Autodesk Inventor part; units mm, degrees
ref_plane "YZ Plane" through (0, 0, 0) normal (1, 0, 0) x (0, 1, 0)
ref_plane "XZ Plane" through (0, 0, 0) normal (0, 1, 0) x (-1, 0, 0)
ref_plane "XY Plane" through (0, 0, 0) normal (0, 0, 1) x (1, 0, 0)
sketch "Sketch1" plane through (0, 0, 0) normal (0, 0, 1) x (1, 0, 0)
  line L0 (-56.0804, 17.6748) -> (23.9196, 17.6748)
  line L1 (23.9196, 17.6748) -> (23.9196, -24.3252)
  line L2 (23.9196, -24.3252) -> (-56.0804, -24.3252)
  line L3 (-56.0804, -24.3252) -> (-56.0804, 17.6748)
  line L4 (-57.3304, 19.1748) -> (25.4196, 19.1748)
  line L5 (25.4196, 19.1748) -> (25.4196, -25.8252)
  line L6 (25.4196, -25.8252) -> (-57.3304, -25.8252)
  line L7 (-57.3304, -25.8252) -> (-57.3304, 19.1748)
  point P0 (0, 0)
  dimension "d0" = 80
  dimension "d1" = 42
  dimension "d2" = 1.5
  dimension "d3" = 1.5
  dimension "d4" = 1.25
  dimension "d5" = 1.5
extrude "Extrusion1" add sketch "Sketch1" along normal blind 24
sketch "Sketch2" plane through (0, 0, 0) normal (0, 0, -1) x (-1, 0, 0)
  line L0 (-25.4196, -25.8252) -> (-25.4196, 19.1748)
  line L1 (57.3304, -25.8252) -> (-25.4196, -25.8252)
  line L2 (-25.4196, 19.1748) -> (57.3304, 19.1748)
  line L3 (57.3304, 19.1748) -> (57.3304, -25.8252)
  line L4 (57.3304, -25.8252) -> (-25.4196, -25.8252)
  line L5 (-25.4196, -25.8252) -> (-25.4196, 19.1748)
  point P0 (0, 0)
extrude "Extrusion2" add sketch "Sketch2" along normal blind 1.2
fillet "Fillet1" radius 2 4 edges at (-57.3304, 19.1748, 11.4) (-57.3304, -25.8252, 11.4) (25.4196, -25.8252, 11.4) (25.4196, 19.1748, 11.4)
sketch "Sketch3" plane through (0, 0, 0) normal (0, 0, 1) x (1, 0, 0)
  line L0 (-56.0804, 17.6748) -> (23.9196, 17.6748)
  line L1 (-45.0804, 17.6748) -> (17.9196, 17.6748)
  line L2 (17.9196, 17.6748) -> (17.9196, -24.8955)
  line L3 (17.9196, -24.8955) -> (-45.0804, -24.8955)
  line L4 (-45.0804, -24.8955) -> (-45.0804, 17.6748)
  line L5 (23.9196, 17.6748) -> (23.9196, -24.3252)
  point P0 (0, 0)
  point P1 (17.9196, 17.6748)
  dimension "d11" = 6
  dimension "d12" = 69
extrude "Extrusion3" cut sketch "Sketch3" against normal blind 1.2
chamfer "Chamfer1" distance 1.2 angle 45 2 edges at (-45.0804, -3.3252, 0) (17.9196, -3.3252, 0)
sketch "Sketch4" plane through (-57.3304, -23.8252, 24) normal (-1, 0, 0) x (0, 0, 1)
  line L0 (-15, 14.5) -> (-20, 14.5)
  line L1 (-20, 14.5) -> (-20, 4.5)
  line L2 (-20, 4.5) -> (-15, 4.5)
  line L3 (-15, 4.5) -> (-15, 14.5)
  line L4 (-24, -0.5) -> (-24, 41.5)
  line L5 (-24, -0.5) -> (0, -0.5)
  point P0 (-24, 23.8252)
  dimension "d18" = 4
  dimension "d19" = 5
  dimension "d20" = 10
  dimension "d21" = 5
extrude "Extrusion4" cut sketch "Sketch4" against normal blind 1.5
sketch "Sketch5" plane through (-57.3304, -23.8252, 24) normal (-1, 0, 0) x (0, 0, 1)
  line L0 (0, 43) -> (-25.2, 43)
  line L1 (-25.2, -2) -> (0, -2)
  line L2 (0, 41) -> (0, 0)
  point P0 (-24, 23.8252)
  point P1 (-3, 33)
  point P2 (-3, 8)
  dimension "d24" = 10
  dimension "d25" = 10
  dimension "d26" = 3
  dimension "d27" = 3
hole "Hole1" at (-57.3304, 9.1748, 21) at (-57.3304, -15.8252, 21) direction (1, 0, 0) diameter 2 depth 10 tip angle 179 countersink diameter 4 countersink angle 90
sketch "Sketch6" plane through (25.4196, -23.8252, 24) normal (1, 0, 0) x (0, 0, -1)
  circle A0 centre (3, 8) radius 1
  circle A1 centre (3, 33) radius 1
  point P0 (24, 23.8252)
hole "Hole2" at (25.4196, -15.8252, 21) at (25.4196, 9.1748, 21) direction (-1, 0, 0) diameter 2 depth 10 tip angle 179 countersink diameter 4 countersink angle 90
sketch "Sketch7" plane through (0, 0, -1.2) normal (0, 0, -1) x (-1, 0, 0)
  line L0 (45.0804, -24.8955) -> (-17.9196, -24.8955)
  line L1 (-17.9196, -24.3252) -> (-17.9196, 17.6748)
  line L2 (45.0804, -24.8955) -> (-17.9196, -24.8955)
  line L3 (-17.9196, -24.8955) -> (-17.9196, -24.3252)
  line L4 (-17.9196, -24.3252) -> (45.0804, -24.3252)
  line L5 (45.0804, -24.3252) -> (45.0804, -24.8955)
  point P0 (0, 0)
extrude "Extrusion5" add sketch "Sketch7" against normal blind 1.5
sketch "Sketch8" plane through (0, 0, -1.2) normal (0, 0, -1) x (-1, 0, 0)
  line L0 (-17.9196, -24.3252) -> (-17.9196, 17.6748)
  line L1 (-23.9196, -24.3252) -> (56.0804, -24.3252)
  line L2 (-17.9196, 17.6748) -> (41.0804, 17.6748)
  line L3 (41.0804, 17.6748) -> (41.0804, -24.3252)
  line L4 (41.0804, -24.3252) -> (-17.9196, -24.3252)
  line L5 (-17.9196, -24.3252) -> (-17.9196, 17.6748)
  line L6 (-23.9196, 17.6748) -> (-23.9196, -24.3252)
  line L7 (46.2804, -24.3252) -> (56.0804, -24.3252)
  line L8 (41.0804, 17.6748) -> (56.0804, 17.6748)
  line L9 (56.0804, 17.6748) -> (56.0804, -24.3252)
  line L10 (56.0804, -24.3252) -> (41.0804, -24.3252)
  line L11 (41.0804, -24.3252) -> (41.0804, 17.6748)
  point P0 (0, 0)
  dimension "d44" = 65
extrude "Extrusion6" add sketch "Sketch8" against normal blind 1.2 contours L3 L8 L9 L1
sketch "Sketch9" plane through (0, 0, -1.2) normal (0, 0, -1) x (-1, 0, 0)
  point P0 (0, 0)
chamfer "Chamfer2" distance 0.5 angle 45 4 edges at (-16.0804, 17.6748, 24) (-56.0804, -3.3252, 24) (-16.0804, -24.3252, 24) (23.9196, -3.3252, 24)
chamfer "Chamfer3" distance 1.2 angle 45 1 edges at (-41.0804, -3.3252, 0)
properties part number "screen cover"
Geometry: final body of the model. Coordinates: model frame, mm. A direction names the side the tool comes from. Coordinates: 2 decimals unless noted, no trailing zeros. Order: outer loops, then holes, each group sorted by start corner. A loop starts at its lowest first (then second) coordinate and runs counter-clockwise, first axis right, second up. Notation, with made-up numbers: (75, -18) -> (116, -18) arc R18 cw to (116, 4) -> close; hole circle Ø8 at (42.25, 88). An arc over 180 degrees is marked (long way). Write each question's results on one line, items separated by ' | '. Start each with the question number.
1) Mould query, pull axis Z, two halves, no side actions, for faces 3 (the flat face through (-15, -25.825, 11)), 4 (the cylindrical face through (24.17, -14.85, 21.22)), 5 (the flat face through (-22, -25, -1.2)). Classes: released by +Z, released by -Z, zero draft, split by the parting line, or undercut.
2) Cut plane C-C, the plane z = 8. Output: boundary loops of the cut face in (x, y), and give its area (3 significant figures).
3) Set-up query: faces 1 (the flat face through (-16, -24.325, 11)), 2 (the flat face through (-17, 19.175, 11)). Return all of +Z, -Z, +X, -X, +Y, -Y with unobstructed straight access to the full face (end or side cutting, diameter ignored); none if empty.
4) Material intervals for line 1 along Y through (x, z) = (-8.5, 17); line 2 along X through (y, z) = (-16, 14); line 3 along Y through (x, z) = (24.25, 21), sorted ascending.
5) First-contact query: pin 1 (3 mm diameter, centred on y = 9.17, z = 21, fed in from +X); pin 2 (0.6 mm diameter, centred on x = -56.5, z = 6.5, fed in from +Y); pin 3 (3 mm diameter, centred on y = -15.83, z = 21, fed in from -X). Flat tips, straight axial feed; report the tip coordinate or a pass-through.
6) Cut plane A-A, the plane x = -10. Output: boundary loops of the cut face in (y, z).
7) Cut plane D-D, the plane z = 14.5. Output: boundary loops of the cut face in (x, y).
Checks:
1) face 3: zero draft | face 4: undercut | face 5: released by -Z
2) outline: (-57.33, -23.83) arc R2 ccw to (-55.33, -25.83) -> (23.42, -25.83) arc R2 ccw to (25.42, -23.83) -> (25.42, 17.17) arc R2 ccw to (23.42, 19.17) -> (-55.33, 19.17) arc R2 ccw to (-57.33, 17.17) -> (-57.33, -9.33) -> (-56.08, -9.33) -> (-56.08, 17.67) -> (23.92, 17.67) -> (23.92, -24.33) -> (-56.08, -24.33) -> (-56.08, -19.33) -> (-57.33, -19.33) -> close | area: 348 mm^2
3) face 1: +Z | face 2: +Z, -Z, +X, -X, +Y
4) line 1: -25.83 to -24.33, 17.67 to 19.17 | line 2: -57.33 to -56.08, 23.92 to 25.42 | line 3: -25.64 to -16.83, -14.83 to 8.17, 10.17 to 18.99
5) pin 1: x = 24.92 | pin 2: y = 18.98 | pin 3: x = -56.84
6) outline: (-25.83, -1.2) -> (-24.33, -1.2) -> (-24.33, 23.5) -> (-24.83, 24) -> (-25.83, 24) -> close; (17.67, -1.2) -> (19.17, -1.2) -> (19.17, 24) -> (18.17, 24) -> (17.67, 23.5) -> close
7) outline: (-57.33, -23.83) arc R2 ccw to (-55.33, -25.83) -> (23.42, -25.83) arc R2 ccw to (25.42, -23.83) -> (25.42, 17.17) arc R2 ccw to (23.42, 19.17) -> (-55.33, 19.17) arc R2 ccw to (-57.33, 17.17) -> close; hole (-56.08, -24.33) -> (23.92, -24.33) -> (23.92, 17.67) -> (-56.08, 17.67) -> close
